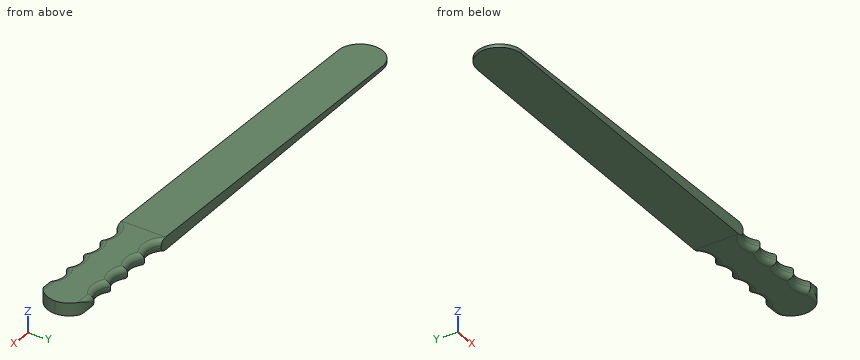
```python
from build123d import *

# Parameters (mm, degrees)
F1_DEPTH = 44.45
F3_DEPTH = 12.701
F4_R     = 5.08
F6_DEPTH = 44.4510001
F8_DEPTH = 12.7


with BuildPart() as f1:
    # F0 (on Front) → F1 (new body)
    with BuildSketch(Plane.XZ):
        Polygon((482.6, 0), (482.6, 6.35), (0, 6.35), (0, 0), (0, -6.35), (482.6, -6.35), align=None)
    extrude(amount=F1_DEPTH)

    # F2 (on face) → F3 (cut, through all)
    with BuildSketch(Plane.XY.offset(6.35)):
        with BuildLine():
            Line((381, 0), (355.6, 0))
            ThreePointArc((355.6, 0), (368.3, -5.08), (381, 0))
        make_face()
        with BuildLine():
            Line((457.2, 0), (431.8, 0))
            ThreePointArc((431.8, 0), (444.5, -5.08), (457.2, 0))
        make_face()
        with BuildLine():
            Line((431.8, 0), (406.4, 0))
            ThreePointArc((406.4, 0), (419.1, -5.08), (431.8, 0))
        make_face()
        with BuildLine():
            Line((406.4, 0), (381, 0))
            ThreePointArc((381, 0), (393.7, -5.08), (406.4, 0))
        make_face()
        with BuildLine():
            ThreePointArc((457.2, -44.45), (444.5, -39.37), (431.8, -44.45))
            Line((431.8, -44.45), (457.2, -44.45))
        make_face()
        with BuildLine():
            ThreePointArc((431.8, -44.45), (419.1, -39.37), (406.4, -44.45))
            Line((406.4, -44.45), (431.8, -44.45))
        make_face()
        with BuildLine():
            ThreePointArc((406.4, -44.45), (393.7, -39.37), (381, -44.45))
            Line((381, -44.45), (406.4, -44.45))
        make_face()
        with BuildLine():
            ThreePointArc((381, -44.45), (368.3, -39.37), (355.6, -44.45))
            Line((355.6, -44.45), (381, -44.45))
        make_face()
    extrude(amount=-F3_DEPTH, mode=Mode.SUBTRACT)

    # F4
    f4_edges = [f1.edges().sort_by_distance(p)[0] for p in [
        (368.3, -39.37, 6.35),
        (393.7, -39.37, 6.35),
        (419.1, -39.37, 6.35),
        (444.5, -39.37, 6.35),
        (444.5, -5.08, 6.35),
        (419.1, -5.08, 6.35),
        (393.7, -5.08, 6.35),
        (368.3, -5.08, 6.35),
        (419.1, -39.37, -6.35),
        (393.7, -39.37, -6.35),
        (368.3, -39.37, -6.35),
        (444.5, -39.37, -6.35),
        (469.9, -44.45, 6.35),
        (469.9, -44.45, -6.35),
        (469.9, 0, 6.35),
        (469.9, 0, -6.35),
        (444.5, -5.08, -6.35),
        (419.1, -5.08, -6.35),
        (393.7, -5.08, -6.35),
        (368.3, -5.08, -6.35),
    ]]
    fillet(f4_edges, radius=F4_R)

    # F5 (on face) → F6 (cut, through all)
    with BuildSketch(Plane.XZ.offset(44.45)):
        Polygon((0, 6.35), (0, 1.5875), (348.9559363111, 6.35), align=None)
        Polygon((348.9559363111, -6.35), (0, -1.5875), (0, -6.35), align=None)
    extrude(amount=-F6_DEPTH, mode=Mode.SUBTRACT)

    # F7 (on Top) → F8 (cut, symmetric)
    with BuildSketch(Plane.XY):
        with BuildLine():
            ThreePointArc((22.225, -44.45), (6.5095517881, -37.9404482119), (0, -22.225))
            Line((0, -22.225), (0, -44.45))
            Line((0, -44.45), (22.225, -44.45))
        make_face()
        with BuildLine():
            ThreePointArc((0, -22.225), (6.5095517881, -6.5095517881), (22.225, 0))
            Line((22.225, 0), (0, 0))
            Line((0, 0), (0, -22.225))
        make_face()
        with BuildLine():
            ThreePointArc((460.375, 0), (476.0904482119, -6.5095517881), (482.6, -22.225))
            Line((482.6, -22.225), (482.6, 0))
            Line((482.6, 0), (460.375, 0))
        make_face()
        with BuildLine():
            ThreePointArc((482.6, -22.225), (476.0904482119, -37.9404482119), (460.375, -44.45))
            Line((460.375, -44.45), (482.6, -44.45))
            Line((482.6, -44.45), (482.6, -22.225))
        make_face()
    extrude(amount=F8_DEPTH, both=True, mode=Mode.SUBTRACT)


solid = f1.part
```
Here's how the part is built. I have some questions about the finished solid (model axes, mm). Give positions to 0.01 mm unless a question says otherwise; leave off trailing zeros. Loops run counter-clockwise (first coordinate to the right, second up) from the corner with the lowest first, then second, coordinate; pieces in that order, holes last. Notation, with made-up numbers: M -16,82 L -2,82 A25 cw -2,95 Z; hole C 30,-24.75 d7. An arc over 180 degrees is marked long. Use one line per item in the form item = value. Start each with the question number.
Q1. If we section it at C-C (x = 55.5): Write out the boundary of the cut face in (y, z).
Q2. If we section it at B-B (x = 324.5): Write out the boundary of the cut face in (y, z).
Q3. I need wall thicknesses on line 1 along X through (y, z) = (-21.5, 1.25); line 2 along X through (y, z) = (-13.5, -1.25); line 3 along Z through (x, y) = (32.5, -34). Which ranges of each line are inside material? Lowest first, please.
Q4. If we section it at A-A (y = -16): Write out the boundary of the cut face in (x, z).
Q5. Will these pins go through, and if not, where does the flat tip stop? pin 1 Ø4 at (x, z) = (245.5, 5) entering from +Y; pin 2 Ø8 at (x, y) = (303, -22) entering from -Z; pin 3 Ø3 at (y, z) = (-37.5, 2) entering from +X; pin 4 Ø5 at (x, y) = (365.5, -40) entering from -Z.
Taken from the geometry:
q1.outline = M -44.45,-2.34 L 0,-2.34 L 0,2.34 L -44.45,2.34 Z
q2.outline = M -44.45,-6.02 L 0,-6.02 L 0,6.02 L -44.45,6.02 Z
q3.line_1 = 0.01 to 482.59
q3.line_2 = 1.78 to 480.82
q3.line_3 = -2.03 to 2.03
q4.outline = M 0.89,-1.6 L 348.96,-6.35 L 481.71,-6.35 L 481.71,6.35 L 348.96,6.35 L 0.89,1.6 Z
q5.pin_1 = 0
q5.pin_2 = -5.78
q5.pin_3 = 477.82
q5.pin_4 = -5.38
